Part model, mm, in its own coordinate system. Give positions to 0.01 mm unless a question says otherwise; leave off trailing zeros. Write each loop counter-clockwise with the first axis right and the second up, starting at its lowest first coordinate (ties: lowest second). Pieces come first, ordered by that corner, then holes.
```python
from build123d import *

# Parameters (mm, degrees)
F1_DEPTH = 1.27


with BuildPart() as f1:
    # F0 (on Front) → F1 (new body)
    with BuildSketch(Plane.XZ):
        with BuildLine():
            Line((3.246805, 57.773859), (-19.613195, 57.773859))
            ThreePointArc((-19.613195, 57.773859), (-21.409247, 57.02991), (-22.153195, 55.233859))
            Line((-22.153195, 55.233859), (-22.153195, -36.206141))
            ThreePointArc((-22.153195, -36.206141), (-21.409247, -38.002193), (-19.613195, -38.746141))
            Line((-19.613195, -38.746141), (46.426805, -38.746141))
            ThreePointArc((46.426805, -38.746141), (48.222856, -38.002193), (48.966805, -36.206141))
            Line((48.966805, -36.206141), (48.966805, 31.477067))
            ThreePointArc((48.966805, 31.477067), (48.222856, 33.273119), (46.426805, 34.017067))
            Line((46.426805, 34.017067), (41.346805, 34.017067))
            ThreePointArc((41.346805, 34.017067), (25.02413, 38.865573), (13.995192, 51.838633))
            ThreePointArc((13.995192, 51.838633), (9.385916, 56.191471), (3.246805, 57.773859))
        make_face()
    extrude(amount=F1_DEPTH)


solid = f1.part
```
1) Saw through at C-C, the plane x = 20. Write the cut outline in (y, z), then the cut area to 3 significant figures.
Answers follow:
outline: (-1.27, -38.75) - (0, -38.75) - (0, 42.98) - (-1.27, 42.98) - close
area: 104 mm2
2) Pin check, flat tip, straight feed: pin 1 Ø10 at (x, z) = (-10, 18) entering from +Y. Stop position of the tip, or through.
Answers follow:
pin 1: stops at y = 0
3) Wall check: L1, parallel to Z at x = 41.5, y = -0.7; L2, parallel to Z at x = 34.5, y = -0.3; L3, parallel to X at y = -0.4, z = 42.5. Give the ranges that are in metal, low to high.
Answers follow:
L1: z = -38.75 to 34.02
L2: z = -38.75 to 34.81
L3: x = -22.15 to 20.48
4) Saw through at B-B, the plane z = 42. Write the cut outline in (x, y), then the cut area to 3 significant figures.
Answers follow:
outline: (-22.15, -1.27) - (21.01, -1.27) - (21.01, 0) - (-22.15, 0) - close
area: 54.8 mm2
5) Saw through at A-A, the plane y = -0.35. Write the cut outline in (x, z), then the cut area to 3 significant figures.
Answers follow:
outline: (-22.15, -36.21) arc R2.54 ccw to (-19.61, -38.75) - (46.43, -38.75) arc R2.54 ccw to (48.97, -36.21) - (48.97, 31.48) arc R2.54 ccw to (46.43, 34.02) - (41.35, 34.02) arc R29.9 cw to (14, 51.84) arc R12.7 ccw to (3.25, 57.77) - (-19.61, 57.77) arc R2.54 ccw to (-22.15, 55.23) - close
area: 6,150 mm2
